Input: part model. Units: mm. Frame: model coordinates. Give positions to 0.01 mm unless a question says otherwise; leave off trailing zeros. Loops run counter-clockwise (first coordinate to the right, second up) from the corner with the lowest first, then second, coordinate; pieces in that order, holes last.
from build123d import *

# Parameters (mm, degrees)
F0_W     = 62.1536839753
F0_H     = 136.7805153131
F1_DEPTH = 2.5
F3_D     = 4.2
F5_D     = 8.5
F5_DEPTH = 17.2
F5_TIP   = 2.5536576309


with BuildPart() as f1:
    # F0 (on Top) → F1 (new body, symmetric)
    with BuildSketch(Plane.XY):
        with Locations((-1.0015358767, -0.7572177634)):
            Rectangle(F0_W, F0_H)
    extrude(amount=F1_DEPTH, both=True)

    # F3 (through all)
    with Locations(Plane.XY.offset(2.5)):
        with Locations((-12.85, -12.898471453), (-12.85, 12.898471453), (12.85, -12.898471453), (12.85, 12.898471453)):
            Hole(F3_D / 2)

    # F5
    with Locations(Plane.XY.offset(2.5)):
        with Locations((-17.0783778643, 52.6330398932), (17.0783778643, 52.6330398932), (17.0783778643, -52.6330398932), (-17.0783778643, -52.6330398932)):
            Hole(F5_D / 2, depth=F5_DEPTH)
            with Locations((0, 0, -(F5_DEPTH + F5_TIP / 2))):  # 118° drill point
                Cone(0, F5_D / 2, F5_TIP, mode=Mode.SUBTRACT)


solid = f1.part
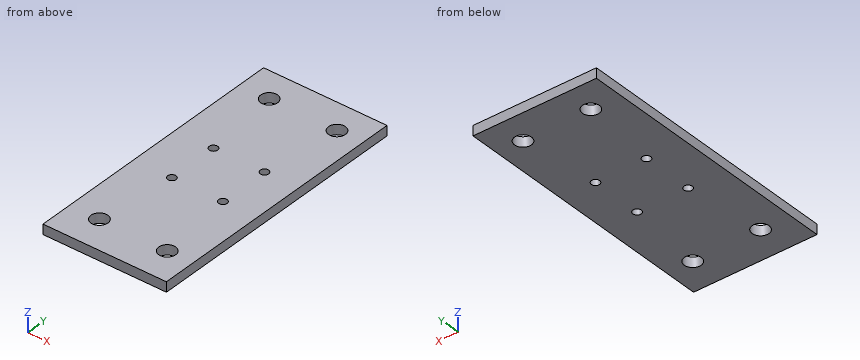
(1) Pin query (flat end, axial travel): pin 1 Ø10 at (x, y) = (17.08, 52.63) entering from +Z. Return the tip coordinate at first contact, or that it passes through.
Values follow:
pin 1: stops at z = 2.5
(2) Cut plane C-C (y = 50.5). Return the cut outline in (x, z).
Values follow:
outline: (-32.08, -2.5) - (-20.75, -2.5) - (-20.75, 2.5) - (-32.08, 2.5) - close; (-13.4, -2.5) - (13.4, -2.5) - (13.4, 2.5) - (-13.4, 2.5) - close; (20.75, -2.5) - (30.08, -2.5) - (30.08, 2.5) - (20.75, 2.5) - close
(3) Cut plane A-A (x = -17). Return the cut outline in (y, z), and give its area (3 significant figures).
Values follow:
outline: (-69.15, -2.5) - (-56.88, -2.5) - (-56.88, 2.5) - (-69.15, 2.5) - close; (-48.38, -2.5) - (48.38, -2.5) - (48.38, 2.5) - (-48.38, 2.5) - close; (56.88, -2.5) - (67.63, -2.5) - (67.63, 2.5) - (56.88, 2.5) - close
area: 599 mm2
(4) Ray query, probe 1 along Y at (x, z) = (-19.5, -2.2); probe 2 along X at (y, z) = (11, 0.15); probe 3 along X at (y, z) = (14.5, 0.3). Return the intervals inside material, ascending.
Values follow:
probe 1: y = -69.15 to -56.13, -49.14 to 49.14, 56.13 to 67.63
probe 2: x = -32.08 to -13.75, -11.95 to 11.95, 13.75 to 30.08
probe 3: x = -32.08 to -14.21, -11.49 to 11.49, 14.21 to 30.08
(5) Cut plane B-B (z = 1.35). Count the separate pieces of the cut face and the enclosed holes in it, and give its area (3 significant figures).
Values follow:
separate pieces: 1
enclosed holes: 8
area: 8,220 mm2
